Read the model definition and answer for the solid it produces. Units are mm, in the model's axes. Round coordinates to 2 decimals unless told otherwise and drop trailing zeros. Order: outer loops, then holes, each group sorted by start corner. A loop starts at its lowest first (then second) coordinate and runs counter-clockwise, first axis right, second up. Notation, with made-up numbers: (-23.75, 58) - (19.25, 58) arc R14 cw to (19.25, 64) - close; hole circle Ø4 at (15, -25). An arc over 180 degrees is marked (long way). Answer as a JSON object with one key per item and string values. Group by question number.
Q1. Given pin 1 Ø12 at (x, z) = (64, 5.5) entering from -Y; pin 2 Ø3 at (x, y) = (54.5, 0.5) entering from -Z; pin 3 Ø1.5 at (x, z) = (-39.5, 2) entering from +Y, each flat-ended and moving along its own axis, determine where each tip first touches the part or whether it passes through.
Q2. A cutting plane is placed at B-B on x = -90. Determine the outline of the cut face in (y, z), and give its area (3 significant figures).
Q3. Consider line 1 (X direction, y = -0.75, z = 3); line 2 (Y direction, x = -42, z = 0.5); line 3 (Y direction, x = 91, z = 8.5). Determine where each line is inside the solid, lowest interval first.
Q4. A cutting plane is placed at A-A on y = -2.25. Determine the outline of the cut face in (x, z).
Q5. A cutting plane is placed at C-C on z = -13. Determine the outline of the cut face in (x, y).
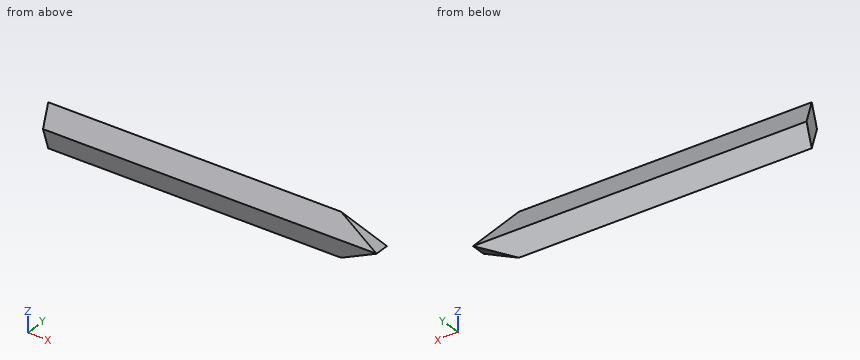
```python
from build123d import *

# Parameters (mm, degrees)
F0_W     = 127
F0_H     = 19.05
F1_DEPTH = 6.35
F3_DEPTH = 298.45
F4_W     = 12.7
F4_H     = 19.05
F5_DEPTH = 324.104


with BuildPart() as f1:
    # F0 (on Front) → F1 (new body, symmetric)
    with BuildSketch(Plane.XZ):
        Polygon((0, 19.05), (-127, 19.05), (-127, -19.05), (0, -19.05), (0, 0), align=None)
        with Locations((63.5, 9.525)):
            Rectangle(F0_W, F0_H)
        Polygon((162.265509367, 0), (127, 19.05), (127, 0), align=None)
        with Locations((63.5, -9.525)):
            Rectangle(F0_W, F0_H)
        Polygon((162.265509367, 0), (127, 0), (127, -19.05), align=None)
    extrude(amount=F1_DEPTH, both=True)

    # F2 (on face) → F3 (cut)
    with BuildSketch(Plane(origin=(-127, 0, 0), x_dir=(0, -1, 0), z_dir=(-1, 0, 0))):
        Polygon((-6.35, 0), (0, 19.05), (-6.35, 19.05), align=None)
        Polygon((0, 19.05), (6.35, 0), (6.35, 19.05), align=None)
    extrude(amount=-F3_DEPTH, mode=Mode.SUBTRACT)

    # F4 (on face) → F5 (cut)
    with BuildSketch(Plane(origin=(-127, 0, 0), x_dir=(0, -1, 0), z_dir=(-1, 0, 0))):
        with Locations((0, -9.525)):
            Rectangle(F4_W, F4_H)
    extrude(amount=-F5_DEPTH, mode=Mode.SUBTRACT)

    # F6: F1 across plane


with BuildPart() as f1_1:
    add(f1.part)
    add(f1.part.mirror(Plane.XY))


solid = f1_1.part
```
Result set:
{
 "1": {"pin 1": "stops at y = -6.35", "pin 2": "stops at z = -19.05", "pin 3": "stops at y = 5.93"},
 "2": {"outline": "(-6.35, 0) - (0, -19.05) - (6.35, 0) - (0, 19.05) - close", "area": "242 mm²"},
 "3": {"line 1": "x = -127 to 156.71", "line 2": "y = -6.18 to 6.18", "line 3": "y = -3.52 to 3.52"},
 "4": {"outline": "(-127, -12.3) - (139.5, -12.3) - (162.27, 0) - (139.5, 12.3) - (-127, 12.3) - close"},
 "5": {"outline": "(-127, -2.02) - (138.2, -2.02) - (138.2, 2.02) - (-127, 2.02) - close"}
}
